Input: part model. Units: mm. Frame: model coordinates. A direction names the side the tool comes from. Give positions to 0.01 mm unless a question says otherwise; leave off trailing zeros. Write each loop counter-clockwise with the first axis right and the second up, starting at its lowest first coordinate (ties: lowest second). Pieces come first, ordered by that corner, then holes.
```python
from build123d import *

# Parameters (mm, degrees)
F0_R     = 38.1
F1_DEPTH = 457.2
F2_R     = 38.1
F3_DEPTH = 457.2
F4_R     = 38.1
F5_DEPTH = 1219.2


with BuildPart() as f1:
    # F0 (on Front) → F1 (new body, symmetric)
    with BuildSketch(Plane.XZ):
        Circle(F0_R)
    extrude(amount=F1_DEPTH, both=True)

    # F2 (on Right) → F3 (join, symmetric)
    with BuildSketch(Plane.YZ):
        Circle(F2_R)
    extrude(amount=F3_DEPTH, both=True)

    # F4 (on Top) → F5 (join)
    with BuildSketch(Plane.XY):
        Circle(F4_R)
    extrude(amount=F5_DEPTH)


solid = f1.part
```
Q1. Pin query (flat end, axial travel): pin 1 (1 mm diameter, centred on x = 23, y = -170, fed in from -Z). Return the tip coordinate at first contact, or that it passes through.
Q2. Material intervals for line 1 along Y through (x, z) = (-4, 988); line 2 along X through (y, z) = (-314, 21); line 3 along Y through (x, z) = (-18.5, 894), sorted ascending.
Q3. Section A-A, the plane z = 0. Return the cut outline in (x, y), then the cut area to 3 significant figures.
Q4. Section B-B, the plane y = 252.5. Return the cut outline in (x, z), then the cut area to 3 significant figures.
Q5. Access query for faces 1 (the cylindrical face through (-8.259, -231.8, -37.194)), 2 (the cylindrical face through (-30.235, -23.183, 614.725)), 3 (the cylindrical face through (-8.259, 225.4, -37.194)). Directions: +Z, -Z, +X, -X, +Y, -Y. A direction counts if a zero-diameter tool reaches every point of the face in a straight line with its end or side. Return the directions, or none.
Solutions:
1. pin 1: stops at z = -30.75
2. line 1: y = -37.89 to 37.89
2. line 2: x = -31.79 to 31.79
2. line 3: y = -33.31 to 33.31
3. outline: (-457.2, -38.1) - (-38.1, -38.1) - (-38.1, -457.2) - (38.1, -457.2) - (38.1, -38.1) - (457.2, -38.1) - (457.2, 38.1) - (38.1, 38.1) - (38.1, 457.2) - (-38.1, 457.2) - (-38.1, 38.1) - (-457.2, 38.1) - close
3. area: 134,000 mm2
4. outline: circle Ø76.2 at (0, 0)
4. area: 4,560 mm2
5. face 1: -Y
5. face 2: +Z
5. face 3: +Y
